Here's how the part is built. I have some questions about the finished solid (model axes, mm). A direction names the side the tool comes from. Coordinates: 2 decimals unless noted, no trailing zeros. Order: outer loops, then holes, each group sorted by start corner. A loop starts at its lowest first (then second) coordinate and runs counter-clockwise, first axis right, second up. Notation, with made-up numbers: (16.5, 56) - (23.5, 56) arc R17 cw to (23.5, 79) - close; hole circle Ø5 at (-22.5, 86.5). An arc over 180 degrees is marked (long way). Use one line per item in the form item = value. Start each with the question number.
from build123d import *

# Parameters (mm, degrees)
SKETCH072_R             = 13.97
PAD035_DEPTH            = 27.94
CHAMFER_ANGLE           = 15
CHAMFER_SIZE            = 2.54
CHAMFER001_SIZE         = 3.81
SKETCH073_R             = 4.445
PAD036_DEPTH            = 2.032
SKETCH074_R             = 1.5875
PAD037_DEPTH            = 14.224
SKETCH099_R             = 1.7526
POCKET026_DEPTH         = 5.08
BODY028_PLACEMENT_ANGLE = 180


with BuildPart() as part:
    # Sketch072 → Pad035 (new body)
    with BuildSketch(Plane.YZ):
        Circle(SKETCH072_R)
    extrude(amount=PAD035_DEPTH)

    # Chamfer
    chamfer_edges = [part.edges().sort_by_distance(p)[0] for p in [
        (0, -13.97, 0),
    ]]
    chamfer_side = part.faces().sort_by_distance((13.97, -13.97, 0))[0]
    chamfer(chamfer_edges, length=CHAMFER_SIZE, angle=CHAMFER_ANGLE, reference=chamfer_side)

    # Chamfer001
    chamfer001_edges = [part.edges().sort_by_distance(p)[0] for p in [
        (27.94, -13.97, 0),
    ]]
    chamfer(chamfer001_edges, length=CHAMFER001_SIZE)

    # Sketch073 (on Face4 of Chamfer001) → Pad036 (join)
    with BuildSketch(Plane.YZ.offset(27.94)):
        Circle(SKETCH073_R)
    extrude(amount=PAD036_DEPTH)

    # Sketch074 (on Face7 of Pad036) → Pad037 (join)
    with BuildSketch(Plane.YZ.offset(29.972)):
        Circle(SKETCH074_R)
    extrude(amount=PAD037_DEPTH)

    # Sketch099 (on Face5 of Pad037) → Pocket026 (cut)
    with BuildSketch(Plane(origin=(0, 0, 0), x_dir=(0, 1, 0), z_dir=(-1, 0, 0))):
        with Locations((0, 9.525)):
            Circle(SKETCH099_R)
        with Locations((8.0645, 0)):
            Circle(SKETCH099_R)
        with Locations((0, -9.525)):
            Circle(SKETCH099_R)
        with Locations((-8.0645, 0)):
            Circle(SKETCH099_R)
    extrude(amount=-POCKET026_DEPTH, mode=Mode.SUBTRACT)


with BuildPart() as part_1:
    # Body028 placement: moved
    add(part.part.moved(Location((-92.202, 0, 0))).rotate(Axis((-92.202, 0, 0), (0, 0, 1)), BODY028_PLACEMENT_ANGLE))


solid = part_1.part
1) Which directions (+Z, -Z, +X, -X, +Y, -Y) give clear straight access to the entire face, cutting with the end or side of a thin tool? Please do faces 4 (the flat face through (-92.202, 0, 0)), 5 (the cylindrical face through (-94.706, 0.228, 7.787)), 6 (the flat face through (-120.142, -4.4, -2.1)).
2) For pin 1 (2 mm diameter, centred on y = -3, z = -9.5, fed in from -X); pin 2 (7 mm diameter, centred on y = -1, z = 2, fed in from -X); pin 3 (2 mm diameter, centred on x = -115.5, y = 7.5, fed in from -Z); pin 4 (1.5 mm diameter, centred on x = -123.5, y = 4, fed in from -Z), each with a flat end and sliding along its axis, tell me the tip position at first contact or that it passes through.
3) If we mould it in two halves opening along Z, with no side actions, what happens to faces 1 (the flat face through (-136.398, 0, 0)), 2 (the flat face through (-97.282, 0, 10)), 3 (the cylindrical face through (-121.14, 0.96, -4.34))? For each: pulls with the +Z half, pulls with the -Z half, needs draft (parallel to the pull), parting line crosses it, or undercut.
4) I need wall thicknesses on probe 1 along Z at (x, y) = (-95.3, 0); probe 2 along Y at (x, z) = (-93.75, 0); probe 3 along X at (y, z) = (5.75, 5.5). Which ranges of each line are inside material? Lowest first, please. Write a range as [from, to].
5) Suppose I cut it at C-C, the plane x = -130. List the corners of the cut face in (y, z) for me (1 decimal), then the cut area to 3 significant figures.
6) Suppose I cut it at B-B, the plane y = 0. List the corners of the cut face in (x, z) for me (1 decimal), then the cut area to 3 significant figures.
7) Suppose I cut it at D-D, the plane x = -115. List the corners of the cut face in (y, z) for me, then the cut area to 3 significant figures.
8) Suppose I cut it at A-A, the plane z = 0. List the corners of the cut face in (x, y) for me (1 decimal), then the cut area to 3 significant figures.
From the geometry:
q1.face_4 = +Z, -Z, +X, +Y, -Y
q1.face_5 = +X
q1.face_6 = -X
q2.pin_1 = -120.14
q2.pin_2 = -136.4
q2.pin_3 = -12.37
q2.pin_4 = through
q3.face_1 = needs draft
q3.face_2 = undercut
q3.face_3 = parting line crosses it
q4.probe_1 = [-13.97, -11.28], [-7.77, 7.77], [11.28, 13.97]
q4.probe_2 = [-13.7, -9.82], [-6.31, 6.31], [9.82, 13.7]
q4.probe_3 = [-120.14, -92.2]
q5.outline = circle Ø3.2 at (0, 0)
q5.area = 7.92 mm2
q6.outline = (-136.4, -1.6) - (-122.2, -1.6) - (-122.2, -4.4) - (-120.1, -4.4) - (-120.1, -10.2) - (-116.3, -14) - (-94.7, -14) - (-92.2, -13.3) - (-92.2, -11.3) - (-97.3, -11.3) - (-97.3, -7.8) - (-92.2, -7.8) - (-92.2, 7.8) - (-97.3, 7.8) - (-97.3, 11.3) - (-92.2, 11.3) - (-92.2, 13.3) - (-94.7, 14) - (-116.3, 14) - (-120.1, 10.2) - (-120.1, 4.4) - (-122.2, 4.4) - (-122.2, 1.6) - (-136.4, 1.6) - close
q6.area = 792 mm2
q7.outline = circle Ø27.94 at (0, 0)
q7.area = 613 mm2
q8.outline = (-136.4, -1.6) - (-122.2, -1.6) - (-122.2, -4.4) - (-120.1, -4.4) - (-120.1, -10.2) - (-116.3, -14) - (-94.7, -14) - (-92.2, -13.3) - (-92.2, -9.8) - (-97.3, -9.8) - (-97.3, -6.3) - (-92.2, -6.3) - (-92.2, 6.3) - (-97.3, 6.3) - (-97.3, 9.8) - (-92.2, 9.8) - (-92.2, 13.3) - (-94.7, 14) - (-116.3, 14) - (-120.1, 10.2) - (-120.1, 4.4) - (-122.2, 4.4) - (-122.2, 1.6) - (-136.4, 1.6) - close
q8.area = 792 mm2
